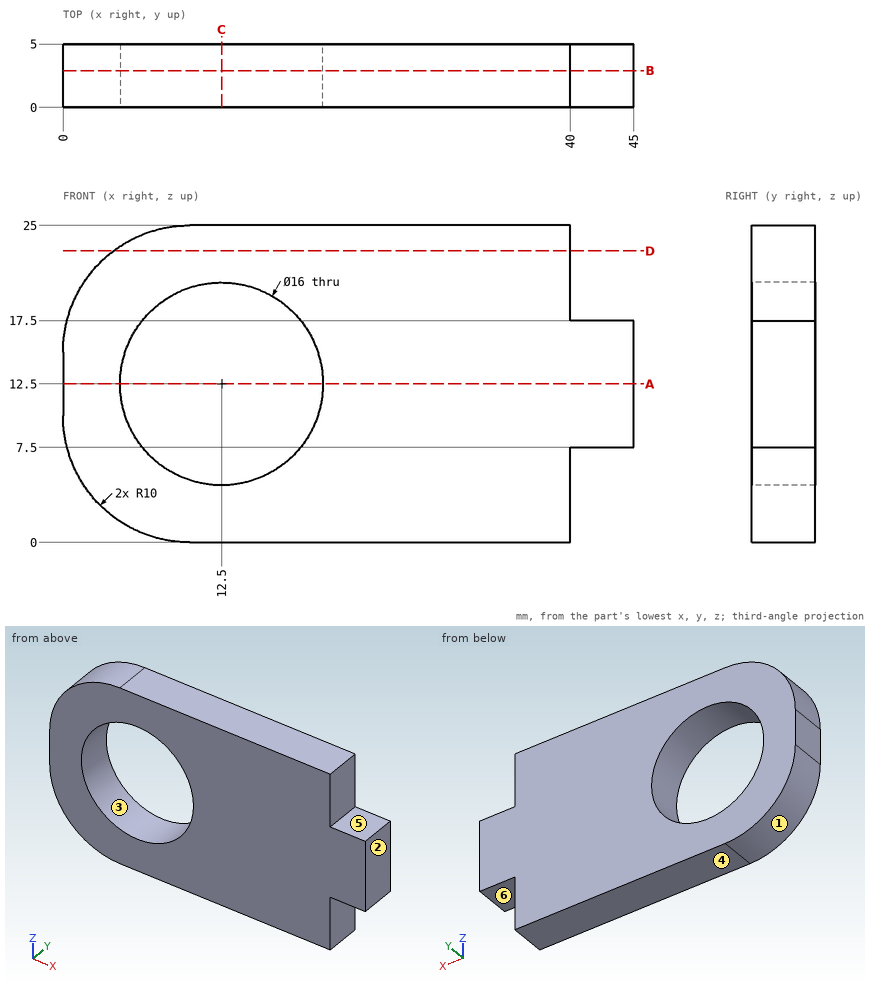
Can you work these out from the drawing? Everything is in mm from the part's minimum corner. A direction names the side the tool comes from. Coordinates: 2 decimals unless noted, no trailing zeros. Write each loop counter-clockwise with the first axis right and the second up, starting at its lowest first coordinate (ties: lowest second). Pieces come first, ordered by that corner, then holes. Notation, with made-up numbers: (13, 24.25) - (28, 24.25) arc R12 cw to (28, 41.25) - close; hole circle Ø10 at (8.5, 75.25). An arc over 180 degrees is marked (long way). One line per item, written item: value.
1) Suppose I cut it at D-D on z = 23. Write out the boundary of the cut face in (x, y), and give its area (3 significant figures).
Model answer:
outline: (4, 0) - (40, 0) - (40, 5) - (4, 5) - close
area: 180 mm²
2) We'd pull the mould along Z, two halves only. Please class the marked faces 1, 2 and 3: pulls with the +Z half, pulls with the -Z half, needs draft (parallel to the pull), parting line crosses it, or undercut.
Model answer:
face 1: pulls with the -Z half
face 2: needs draft
face 3: undercut
3) I'm going to push flat-ended pins straight in: P1, Ø2.5, axis at x = 41.5, y = 3.5, coming from the +Z side; P2, Ø2.5, axis at x = 42.5, y = 1.5, coming from the -Z side. Where does each tip first touch, or does it pass through?
Model answer:
P1: stops at z = 17.5
P2: stops at z = 7.5
4) Suppose I cut it at C-C on x = 12.5. Write out the boundary of the cut face in (y, z), and give its area (3 significant figures).
Model answer:
outline: (0, 0) - (5, 0) - (5, 4.5) - (0, 4.5) - close; (0, 20.5) - (5, 20.5) - (5, 25) - (0, 25) - close
area: 45.0 mm²
5) Suppose I cut it at A-A on z = 12.5. Write out the boundary of the cut face in (x, y), and give its area (3 significant figures).
Model answer:
outline: (0, 0) - (4.5, 0) - (4.5, 5) - (0, 5) - close; (20.5, 0) - (45, 0) - (45, 5) - (20.5, 5) - close
area: 145 mm²
6) Suppose I cut it at B-B on y = 2.9. Write out the boundary of the cut face in (x, z), and give its area (3 significant figures).
Model answer:
outline: (0, 10) arc R10 ccw to (10, 0) - (40, 0) - (40, 7.5) - (45, 7.5) - (45, 17.5) - (40, 17.5) - (40, 25) - (10, 25) arc R10 ccw to (0, 15) - close; hole circle Ø16 at (12.5, 12.5)
area: 806 mm²
7) I need wall thicknesses on line 1 along Z through (x, y) = (12.5, 1.9); line 2 along Z through (x, y) = (41.5, 1.7); line 3 along X through (y, z) = (2.75, 9). Which ranges of each line are inside material? Lowest first, please.
Model answer:
line 1: z = 0 to 4.5, 20.5 to 25
line 2: z = 7.5 to 17.5
line 3: x = 0.05 to 5.31, 19.69 to 45
8) On a 3-axis mill with a long thin cutter (end or side, diameter ignored), from which of +Z, -Z, +X, -X, +Y, -Y can I reach the whole of each face in a straight line? I mean the marked faces 4, 5 and 6. Say none if no direction works.
Model answer:
face 4: -Z, +X, -X, +Y, -Y
face 5: +Z, +X, +Y, -Y
face 6: -Z, +X, +Y, -Y
